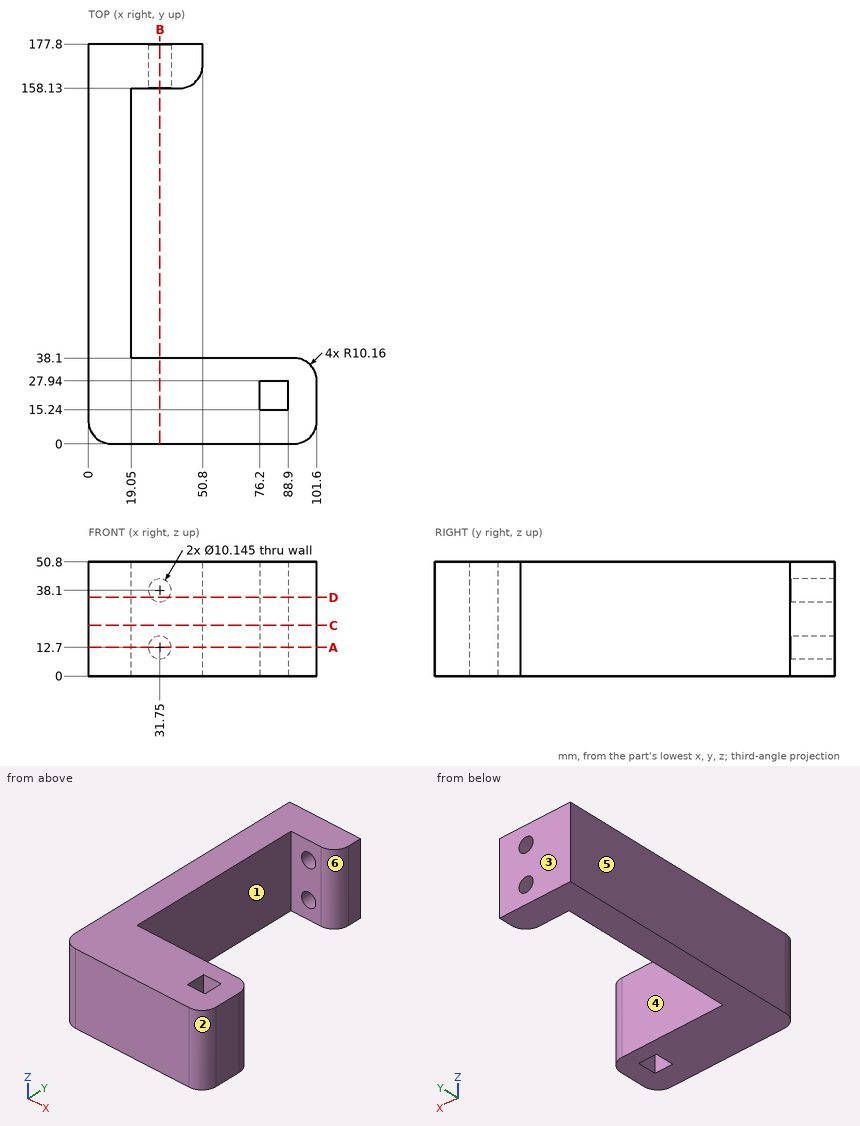
Answer from the drawing. Dimensions are ordinates in mm from the lowest x, y and z of the part. A direction names the side the tool comes from. Coordinates: 2 decimals unless noted, no trailing zeros. Write each loop counter-clockwise with the first axis right and the second up, starting at its lowest first coordinate (ties: lowest second). Pieces come first, ordered by that corner, then holes. Notation, with made-up numbers: (82, -14.75) -> (117, -14.75) arc R30 cw to (117, 12.25) -> close; hole circle Ø11 at (57.25, 46.25). An arc over 180 degrees is marked (long way). One line per question, with ' | ' between items.
1. Straight lines are drawn through the part: line 1 (X direction, y = 167.5, z = 38.1); line 2 (Y direction, x = 87, z = 21); line 3 (Y direction, x = 41.5, z = 30.5). For each, find the intervals that lie inside material, in ascending order.
Verdict:
line 1: x = 0 to 26.68, 36.82 to 50.77 | line 2: y = 0 to 15.24, 27.94 to 38.1 | line 3: y = 0 to 38.1, 158.17 to 177.8
2. Section B-B (x = 31.75) is taken. Determine the outline of the cut face in (y, z).
Verdict:
outline: (0, 0) -> (38.1, 0) -> (38.1, 50.8) -> (0, 50.8) -> close; (158.13, 0) -> (177.8, 0) -> (177.8, 7.63) -> (158.13, 7.63) -> close; (158.13, 17.77) -> (177.8, 17.77) -> (177.8, 33.03) -> (158.13, 33.03) -> close; (158.13, 43.17) -> (177.8, 43.17) -> (177.8, 50.8) -> (158.13, 50.8) -> close
3. For a pull along Y with two mould halves and no side action, classify the marked faces 3, 4, 5 and 6 as released by +Y, released by -Y, zero draft, split by the parting line, or undercut.
Verdict:
face 3: released by +Y | face 4: undercut | face 5: zero draft | face 6: undercut
4. Given pin 1 Ø2 at (x, y) = (19, 49.5) entering from -Z; pin 2 Ø10.5 at (y, z) = (173, 22.5) entering from +X; pin 3 Ø4 at (x, z) = (84, 35.5) entering from +Y; pin 4 Ø3 at (y, z) = (50, 31.5) entering from +X, each flat-ended and moving along its own axis, determine where each tip first touches the part or whether it passes through.
Verdict:
pin 1: stops at z = 0 | pin 2: stops at x = 50.8 | pin 3: stops at y = 38.1 | pin 4: stops at x = 19.05
5. Section A-A (z = 12.7) is taken. Determine the outline of the cut face in (x, y).
Verdict:
outline: (0, 10.16) arc R10.16 ccw to (10.16, 0) -> (91.44, 0) arc R10.16 ccw to (101.6, 10.16) -> (101.6, 27.94) arc R10.16 ccw to (91.44, 38.1) -> (19.05, 38.1) -> (19.05, 158.13) -> (26.68, 158.13) -> (26.68, 177.8) -> (0, 177.8) -> close; (36.82, 158.13) -> (40.64, 158.13) arc R10.16 ccw to (50.8, 168.29) -> (50.8, 177.8) -> (36.82, 177.8) -> close; hole (76.2, 15.24) -> (88.9, 15.24) -> (88.9, 27.94) -> (76.2, 27.94) -> close
6. Section C-C (z = 22.5) is taken. Determine the outline of the cut face in (x, y), and give its area (3 significant figures).
Verdict:
outline: (0, 10.16) arc R10.16 ccw to (10.16, 0) -> (91.44, 0) arc R10.16 ccw to (101.6, 10.16) -> (101.6, 27.94) arc R10.16 ccw to (91.44, 38.1) -> (19.05, 38.1) -> (19.05, 158.13) -> (40.64, 158.13) arc R10.16 ccw to (50.8, 168.29) -> (50.8, 177.8) -> (0, 177.8) -> close; hole (76.2, 15.24) -> (88.9, 15.24) -> (88.9, 27.94) -> (76.2, 27.94) -> close | area: 6,910 mm^2
7. Which of the six approach directions +Z, -Z, +X, -X, +Y, -Y give full straight-line access (tool end or side, diameter ignored) to the marked faces 1 and 2?
Verdict:
face 1: +Z, -Z, +X | face 2: +Z, -Z, +X, -Y
8. Section D-D (z = 35) is taken. State how many separate pieces and enclosed holes the cut face has, and give its area (3 significant figures).
Verdict:
separate pieces: 2 | enclosed holes: 1 | area: 6,750 mm^2
